from build123d import *

# Parameters (mm, degrees)
F0_W     = 425
F0_H     = 584
F1_DEPTH = 6.35
F2_D     = 6.8
F3_D     = 34.5948


with BuildPart() as f1:
    # F0 (on Front) → F1 (new body)
    with BuildSketch(Plane.XZ):
        Rectangle(F0_W, F0_H)
    extrude(amount=F1_DEPTH)

    # F2 (through all)
    with Locations(Plane(origin=(0, 0, 0), x_dir=(1, 0, 0), z_dir=(0, 1, 0))):
        with Locations((-180, -230), (-180, 230), (180, 230), (180, -230)):
            Hole(F2_D / 2)

    # F3 (through all)
    with Locations(Plane(origin=(0, 0, 0), x_dir=(1, 0, 0), z_dir=(0, 1, 0))):
        with Locations((-154.5, -50.8), (-154.5, 0), (-154.5, 50.8)):
            Hole(F3_D / 2)


solid = f1.part
Work out the finished part from the listing and answer in its coordinate system (mm). Coordinates: 2 decimals unless noted, no trailing zeros. Loops run counter-clockwise (first coordinate to the right, second up) from the corner with the lowest first, then second, coordinate; pieces in that order, holes last. Notation, with made-up numbers: (1, -30) -> (7, -30) arc R16 ccw to (7, -4) -> close; hole circle Ø10 at (66.5, -29). An arc over 180 degrees is marked (long way). Answer as CSV lines item,"result".
1) The part is cut by section B-B (z = -50.8). Give the vertices of the cut face in (x, y).
A:
outline,"(-212.5, -6.35) -> (-171.8, -6.35) -> (-171.8, 0) -> (-212.5, 0) -> close; (-137.2, -6.35) -> (212.5, -6.35) -> (212.5, 0) -> (-137.2, 0) -> close"
2) The part is cut by section A-A (x = -154.5). Give the vertices of the cut face in (y, z), and give its area (3 significant figures).
A:
outline,"(-6.35, -292) -> (0, -292) -> (0, -68.1) -> (-6.35, -68.1) -> close; (-6.35, -33.5) -> (0, -33.5) -> (0, -17.3) -> (-6.35, -17.3) -> close; (-6.35, 17.3) -> (0, 17.3) -> (0, 33.5) -> (-6.35, 33.5) -> close; (-6.35, 68.1) -> (0, 68.1) -> (0, 292) -> (-6.35, 292) -> close"
area,"3,050 mm²"
3) Straight lines are drawn through the part: probe 1 along X at (y, z) = (-2.5, -230); probe 2 along Z at (x, y) = (-154.5, -3.5); probe 3 along Z at (x, y) = (-180, -1.5). For each, find the intervals that lie inside material, in ascending order.
A:
probe 1,"x = -212.5 to -183.4, -176.6 to 176.6, 183.4 to 212.5"
probe 2,"z = -292 to -68.1, -33.5 to -17.3, 17.3 to 33.5, 68.1 to 292"
probe 3,"z = -292 to -233.4, -226.6 to 226.6, 233.4 to 292"
4) A flat-ended cylindrical pin translates along its axis: pin 1 (11 mm diameter, centred on x = -180, z = 230, fed in from +Y). Find the tip coordinate at first contact, or state that the pin passes through.
A:
pin 1,"stops at y = 0"
